Work out the finished part from the listing and answer in its coordinate system (mm). A direction names the side the tool comes from. Round coordinates to 2 decimals unless told otherwise and drop trailing zeros. Write each loop counter-clockwise with the first axis right and the second up, starting at its lowest first coordinate (ties: lowest second). Pieces come first, ordered by that corner, then holes.
1. Flat-ended cylindrical pins translate along their axes: pin 1 Ø1 at (x, y) = (2, -1.5) entering from -Z; pin 2 Ø0.5 at (y, z) = (0, 0) entering from -X; pin 3 Ø2 at (y, z) = (-0.5, -0.5) entering from -X. Find the tip coordinate at first contact, or state that the pin passes through.
2. A tool of negligible diameter and unlimited length cuts with its end or side. For faces 1 (the face through (-2, 1.2, 0)), 2 (the face through (0, 2, 0)), 3 (the face through (-1.408, 0.491, -0.867)), from which of +Z, -Z, +X, -X, +Y, -Y can it reach the whole face along a straight path? Write none if from no direction.
3. Find section C-C (y = -1.75). Write down the section's boundary in (x, z).
4. Find section A-A (z = 0). Write down the section's boundary in (x, y), and give its area (3 significant figures).
5. Determine the mould class of faces 4 (the face through (-0.986, -0.596, -2.685)), 5 (the face through (-0.6, 0, 0)), 6 (the face through (6, 0, 0)) for opening direction Y: pulls with the +Y half, pulls with the -Y half, needs draft (parallel to the pull), parting line crosses it, or undercut.
6. Find section D-D (x = -0.5). Write down the section's boundary in (y, z), and give its area (3 significant figures).
7. Find section B-B (x = 0.5). Write down the section's boundary in (y, z).
8. Straight lines are drawn through the part: probe 1 along Y at (x, z) = (-1, 0.1); probe 2 along X at (y, z) = (-0.3, -0.7); probe 3 along Z at (x, y) = (1.25, 0). For each, find the intervals that lie inside material, in ascending order.
Autodesk Inventor part; units mm, degrees
ref_plane "YZ Plane" through (0, 0, 0) normal (1, 0, 0) x (0, 1, 0)
ref_plane "XZ Plane" through (0, 0, 0) normal (0, 1, 0) x (-1, 0, 0)
ref_plane "XY Plane" through (0, 0, 0) normal (0, 0, 1) x (1, 0, 0)
sketch "スケッチ1" plane through (0, 0, 0) normal (0, 0, 1) x (1, 0, 0)
  line L0 (0, 0) -> (6, 0)
  line L1 (6, 0) -> (6, 1.5)
  line L2 (6, 1.5) -> (0, 1.5)
  line L3 (0, 1.5) -> (0, 0)
  line L4 (0, 0) -> (0, 2.75)
  line L5 (0, 0) -> (-2, 0)
  line L6 (-2, 0) -> (0, 0)
  line L7 (-2, 0) -> (-2, 1.15)
  line L8 (0, 0) -> (-2, 0)
  line L9 (-2, 0) -> (-2, 2.75)
  line L10 (-2, 2.75) -> (0, 2.75)
  line L11 (0, 2.75) -> (0, 0)
  dimension "d0" = 1.5
  dimension "d1" = 6
  dimension "d3" = 2
  dimension "d4" = 2.75
  dimension "d5" = 1.15
revolve "回転1" add sketch "スケッチ1" angle 360 about axis through (-2, 0, 0) along (1, 0, 0)
thread "ねじ1"
sketch "スケッチ2" plane through (-2, 0, 0) normal (-1, 0, 0) x (0, 0, 1)
  circle A0 centre (0, 0) radius 1.15
  line L0 (-0.575, 0.9959) -> (0.575, 0.9959)
  line L1 (0.575, 0.9959) -> (1.15, 0)
  line L2 (1.15, 0) -> (0.575, -0.9959)
  line L3 (0.575, -0.9959) -> (-0.575, -0.9959)
  line L4 (-0.575, -0.9959) -> (-1.15, 0)
  line L5 (-1.15, 0) -> (-0.575, 0.9959)
  dimension "d10" = 1.15
  dimension "d11" = 1.9919
extrude "押し出し1" cut sketch "スケッチ2" against normal blind 1.4 contours L2 L3 L4 L5 L0 L1
fillet "フィレット1" radius 0.2 6 edges at (-0.6, 0.9959, 0) (-0.6, 0.498, 0.8625) (-0.6, 0.498, -0.8625) (-0.6, -0.498, -0.8625) (-0.6, -0.9959, 0) (-0.6, -0.498, 0.8625)
fillet "フィレット2" radius 0.1 1 edges at (0, -1.5, 0)
fillet "フィレット3" radius 0.1 1 edges at (6, -1.5, 0)
properties part number "ネジキャップM3L6" material "鋼"
Worked answers:
1. pin 1: stops at z = -1.12
1. pin 2: stops at x = -0.6
1. pin 3: stops at x = -2
2. face 1: +Z, -Z, -X, +Y, -Y
2. face 2: +X
2. face 3: -X
3. outline: (-2, -2.12) - (0, -2.12) - (0, 2.12) - (-2, 2.12) - close
4. outline: (-2, -2.75) - (0, -2.75) - (0, -1.6) arc R0.1 cw to (0.1, -1.5) - (5.9, -1.5) arc R0.1 ccw to (6, -1.4) - (6, 1.4) arc R0.1 ccw to (5.9, 1.5) - (0.1, 1.5) arc R0.1 cw to (0, 1.6) - (0, 2.75) - (-2, 2.75) - (-2, 1) - (-0.8, 1) arc R0.2 cw to (-0.6, 0.8) - (-0.6, -0.8) arc R0.2 cw to (-0.8, -1) - (-2, -1) - close
4. area: 26.2 mm2
5. face 4: parting line crosses it
5. face 5: undercut
5. face 6: needs draft
6. outline: circle Ø5.5 at (0, 0)
6. area: 23.8 mm2
7. outline: circle Ø3 at (0, 0)
8. probe 1: y = -2.75 to -1, 1 to 2.75
8. probe 2: x = -0.6 to 6
8. probe 3: z = -1.5 to 1.5
